from build123d import *

# Parameters (mm, degrees)
F0_W     = 55.4736
F0_H     = 43.2816
F1_DEPTH = 12.7
F2_W     = 48.768
F2_H     = 36.576
F3_DEPTH = 10.16
F4_R     = 3.81
F5_DEPTH = 3.81


# Not quite as in the source:
# - a feature names something its author has since deleted; it is built from what else it names


with BuildPart() as f1:
    # F0 (on Top) → F1 (new body)
    with BuildSketch(Plane.XY):
        Rectangle(F0_W, F0_H)
    extrude(amount=F1_DEPTH)

    # F2 (on face) → F3 (cut)
    with BuildSketch(Plane.XY.offset(12.7)):
        Rectangle(F2_W, F2_H)
    extrude(amount=-F3_DEPTH, mode=Mode.SUBTRACT)

    # F4 (on face) → F5 (join)
    with BuildSketch(Plane(origin=(0, 0, 0), x_dir=(1, 0, 0), z_dir=(0, 0, -1))):
        with Locations((15.24, -10.16)):
            Circle(F4_R)
        with Locations((-15.24, -10.16)):
            Circle(F4_R)
        with Locations((15.24, 10.16)):
            Circle(F4_R)
        with Locations((-15.24, 10.16)):
            Circle(F4_R)
    extrude(amount=F5_DEPTH)


solid = f1.part
Read the model definition and answer for the solid it produces. Units are mm, in the model's axes. A direction names the side the tool comes from. Coordinates: 2 decimals unless noted, no trailing zeros. Loops run counter-clockwise (first coordinate to the right, second up) from the corner with the lowest first, then second, coordinate; pieces in that order, holes last. Notation, with made-up numbers: (-32, 26) -> (18, 26) arc R14 cw to (18, 37) -> close; hole circle Ø7 at (74.25, 9.25). An arc over 180 degrees is marked (long way). Write item = value, one per line. Start each with the question number.
1) The mould has two halves that part along Y. Classify faces 4 (the face through (0, -21.641, 6)), 5 (the face through (27.737, 0, 6)), 6 (the face through (-24.384, 0, 8)): pulls with the +Y half, pulls with the -Y half, needs draft (parallel to the pull), parting line crosses it, or undercut.
2) The part is cut by section B-B, the plane x = 2.5. Determine the outline of the cut face in (y, z), plus the area to 3 significant figures.
3) Given P1, Ø5, axis at x = -20.5, y = 0.5, coming from the +Z side, flat-ended and moving along its own axis, determine where the tip first touches the part or whether it passes through.
4) The part is cut by section D-D, the plane z = -2. Determine the outline of the cut face in (x, y).
5) The part is cut by section A-A, the plane z = 11.5. Determine the outline of the cut face in (x, y).
6) For faces 1 (the face through (0, 18.288, 8)), 2 (the face through (0, 19, 12.7)), 3 (the face through (-11.606, 9.016, -1.878)), determine the directions among +Z, -Z, +X, -X, +Y, -Y from which every point of the face is accessible in a straight line to the end or side of a thin tool.
7) The part is cut by section C-C, the plane y = -10.16. Determine the outline of the cut face in (x, z), plus the area to 3 significant figures.
8) Find the intervals of material crossed by L1, parallel to X at y = 7, z = 7.5; L2, parallel to Y at x = -7, z = 7; L3, parallel to Z at x = -7, y = -2, in increasing order. Write a range as from..to.
Result:
q1.face_4 = pulls with the -Y half
q1.face_5 = needs draft
q1.face_6 = undercut
q2.outline = (-21.64, 0) -> (21.64, 0) -> (21.64, 12.7) -> (18.29, 12.7) -> (18.29, 2.54) -> (-18.29, 2.54) -> (-18.29, 12.7) -> (-21.64, 12.7) -> close
q2.area = 178 mm²
q3.P1 = 2.54
q4.outline = circle Ø7.62 at (-15.24, -10.16); circle Ø7.62 at (-15.24, 10.16); circle Ø7.62 at (15.24, -10.16); circle Ø7.62 at (15.24, 10.16)
q5.outline = (-27.74, -21.64) -> (27.74, -21.64) -> (27.74, 21.64) -> (-27.74, 21.64) -> close; hole (-24.38, -18.29) -> (24.38, -18.29) -> (24.38, 18.29) -> (-24.38, 18.29) -> close
q6.face_1 = +Z
q6.face_2 = +Z, +X, -X, +Y, -Y
q6.face_3 = -Z
q7.outline = (-27.74, 0) -> (-19.05, 0) -> (-19.05, -3.81) -> (-11.43, -3.81) -> (-11.43, 0) -> (11.43, 0) -> (11.43, -3.81) -> (19.05, -3.81) -> (19.05, 0) -> (27.74, 0) -> (27.74, 12.7) -> (24.38, 12.7) -> (24.38, 2.54) -> (-24.38, 2.54) -> (-24.38, 12.7) -> (-27.74, 12.7) -> close
q7.area = 267 mm²
q8.L1 = -27.74..-24.38, 24.38..27.74
q8.L2 = -21.64..-18.29, 18.29..21.64
q8.L3 = 0..2.54
